Geometry check sheet. Reference: the model listing, model coordinates, mm. Face numbers are marked on the shaded views. Round coordinates to 2 decimals unless told otherwise and drop trailing zeros. Write each loop counter-clockwise with the first axis right and the second up, starting at its lowest first coordinate (ties: lowest second). Pieces come first, ordered by that corner, then holes.
Item 1: Cross-section at A-A (x = 8). Enter the section's corners in (y, z).
Item 2: Cross-section at C-C (z = 8). Enter the section's corners in (x, y), then the cut area to 3 significant figures.
Item 3: Cross-section at B-B (y = 4.25). Enter the section's corners in (x, z).
Item 4: Draft check along Z on the marked faces 1, 2, 3 and 4. Enter one of: pulls with the +Z half, pulls with the -Z half, needs draft (parallel to the pull), parting line crosses it, or undercut.
Item 5: Scan lines: probe 1 along X at (y, z) = (5.25, 8); probe 2 along X at (y, z) = (4, 8.5); probe 3 along Z at (x, y) = (26.5, 1). Record each from-to range of solid material in increasing order.
Item 6: Cross-section at D-D (z = 2.5). Enter the section's corners in (x, y), then the cut area to 3 significant figures.
from build123d import *

# Parameters (mm, degrees)
SKETCH1_R           = 2.6
BOSS_EXTRUDE1_DEPTH = 6.4
FILLET1_R           = 6
FILLET2_R           = 10
FILLET3_R           = 0.4
FILLET4_R           = 2


with BuildPart() as part:
    # Sketch1 → Boss-Extrude1 (new body)
    with BuildSketch(Plane(origin=(0, 0, 0), x_dir=(1, 0, 0), z_dir=(0, 1, 0))):
        Polygon((36, -13), (36, 0), (0, 0), (0, -5), (-13, -16.5), (-1.455462178, -16.5), (30, -16.5), align=None)
        with Locations(Location((28, -8, 0), (0, 0, 270))):
            Circle(SKETCH1_R, mode=Mode.SUBTRACT)
        with Locations(Location((8, -8, 0), (0, 0, 270))):
            Circle(SKETCH1_R, mode=Mode.SUBTRACT)
    extrude(amount=BOSS_EXTRUDE1_DEPTH)

    # Fillet1
    # the kernel refuses this fillet: 6 mm, written as the material it takes off along each edge
    with BuildSketch(Plane(origin=(30, -4.05523712, 16.5), x_dir=(-1, 0, 0), z_dir=(0, 1, 0))) as fillet1_piece_1:
        with BuildLine():
            CenterArc((FILLET1_R * 0.27034914135, -FILLET1_R), FILLET1_R, 90, 30.256437164)
            Line((-FILLET1_R * 0.233521884174, -FILLET1_R * 0.136221099102), (-FILLET1_R * 0.243599304685, -FILLET1_R * 0.118945521084))
            Line((-FILLET1_R * 0.243599304685, -FILLET1_R * 0.118945521084), (-FILLET1_R * 0.005406982827, FILLET1_R * 0.02))
            Line((-FILLET1_R * 0.005406982827, FILLET1_R * 0.02), (FILLET1_R * 0.27034914135, FILLET1_R * 0.02))
            Line((FILLET1_R * 0.27034914135, FILLET1_R * 0.02), (FILLET1_R * 0.27034914135, 0))
        make_face()
    extrude(amount=14.51047424, mode=Mode.SUBTRACT)
    with BuildSketch(Plane(origin=(36, -15, 0), x_dir=(0, 0, 1), z_dir=(0, 1, 0))) as fillet1_piece_2:
        with BuildLine():
            CenterArc((FILLET1_R, -FILLET1_R), FILLET1_R, 90, 90)
            Line((0, -FILLET1_R), (-FILLET1_R * 0.02, -FILLET1_R))
            Line((-FILLET1_R * 0.02, -FILLET1_R), (-FILLET1_R * 0.02, FILLET1_R * 0.02))
            Line((-FILLET1_R * 0.02, FILLET1_R * 0.02), (FILLET1_R, FILLET1_R * 0.02))
            Line((FILLET1_R, FILLET1_R * 0.02), (FILLET1_R, 0))
        make_face()
    extrude(amount=36.4, mode=Mode.SUBTRACT)
    with BuildSketch(Plane(origin=(0, -14.790199458, 0), x_dir=(0, 0, 1), z_dir=(0, 1, 0))) as fillet1_piece_3:
        with BuildLine():
            CenterArc((6, 5.916079783), FILLET1_R, 180, 80.405931773)
            Line((0, 5.916079783), (-0.12, 5.916079783))
            Line((-0.12, 5.916079783), (-0.12, 0))
            Line((-0.12, 0), (0, -0.12))
            ThreePointArc((0, -0.12), (2.5, -0.12), (4.98, -0.118321596))
            Line((4.98, -0.118321596), (5, 0))
        make_face()
    extrude(amount=35.980398916, mode=Mode.SUBTRACT)

    # Fillet2
    fillet2_edges = [part.edges().sort_by_distance(p)[0] for p in [
        (0, 3.2, 5),
    ]]
    fillet(fillet2_edges, radius=FILLET2_R)

    # Fillet3
    fillet3_edges = [part.edges().sort_by_distance(p)[0] for p in [
        (-13, 3.2, 16.5),
    ]]
    fillet(fillet3_edges, radius=FILLET3_R)

    # Fillet4
    fillet4_edges = [part.edges().sort_by_distance(p)[0] for p in [
        (36, 3.2, 13),
    ]]
    fillet(fillet4_edges, radius=FILLET4_R)


solid = part.part
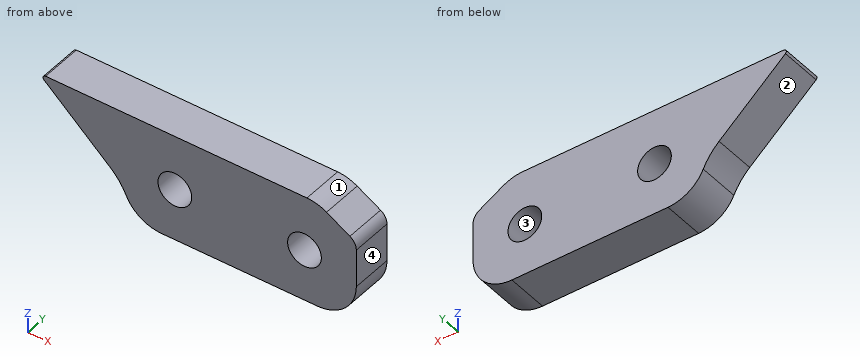
Resolved:
1. outline: (0, 0) - (6.4, 0) - (6.4, 5.4) - (0, 5.4) - close; (0, 10.6) - (6.4, 10.6) - (6.4, 16.5) - (0, 16.5) - close
2. outline: (-3.39, 0) - (5.4, 0) - (5.4, 6.4) - (-3.39, 6.4) - close; (10.6, 0) - (25.4, 0) - (25.4, 6.4) - (10.6, 6.4) - close; (30.6, 0) - (36, 0) - (36, 6.4) - (30.6, 6.4) - close
2. area: 186 mm2
3. outline: (-12.21, 15.8) - (-1.96, 6.74) arc R10 cw to (0.48, 3.47) arc R6 ccw to (5.92, 0) - (30, 0) arc R6 ccw to (36, 6) - (36, 11.85) arc R2 ccw to (35.01, 13.58) - (31.4, 15.68) arc R6 ccw to (28.38, 16.5) - (-11.94, 16.5) arc R0.4 ccw to start; hole circle Ø5.2 at (8, 8); hole circle Ø5.2 at (28, 8)
4. face 1: pulls with the +Z half
4. face 2: pulls with the -Z half
4. face 3: undercut
4. face 4: needs draft
5. probe 1: x = -3.39 to 5.4, 10.6 to 25.4, 30.6 to 36
5. probe 2: x = -3.96 to 5.45, 10.55 to 25.45, 30.55 to 36
5. probe 3: z = 0 to 5.88, 10.12 to 16.5
6. outline: (1.04, 0) - (34.87, 0) - (34.87, 6.4) - (1.04, 6.4) - close
6. area: 217 mm2
